Input: part model. Units: mm. Frame: model coordinates. A direction names the side the tool comes from. Give positions to 0.01 mm unless a question says otherwise; leave off trailing zeros. Write each loop counter-clockwise with the first axis right and the second up, starting at its lowest first coordinate (ties: lowest second). Pieces come first, ordered by that corner, then holes. Notation, with made-up numbers: (-29, -12.75) - (-1, -12.75) arc R34 cw to (-1, 21.25) - close; hole circle Ø4 at (10.5, 38). An arc over 180 degrees is marked (long way). Use a Markdown table: item, result. Add a question column.
1. Section query C-C, the plane y = -7. Return loops of the section in (x, z), plus the area to 3 significant figures.
2. Section query D-D, the plane x = -46. Return loops of the section in (y, z).
3. Pin query (flat end, axial travel): pin 1 (9.5 mm diameter, centred on x = -5, y = -6, fed in from +Z); pin 2 (10 mm diameter, centred on x = 0, z = -234.95, fed in from -Y). Return the tip coordinate at first contact, or that it passes through.
4. Material intervals for probe 1 along Z at (x, y) = (0, -16); probe 2 along Y at (x, z) = (-32, 244); probe 3 along Z at (x, y) = (12, -2), sorted ascending.
5. Mould query, pull axis X, two halves, no side actions, for faces 1 (the flat face through (-1, -19, -279.4)), 2 (the cylindrical face through (-1.38, -19.32, -241.15)), 3 (the flat face through (63.5, -19, -4)). Classes: released by +X, released by -X, zero draft, split by the parting line, or undercut.
6. Set-up query: faces 4 (the flat face through (-1, -9, 152.4)), 5 (the flat face through (-63.5, -19, -4)). Return all of +Z, -Z, +X, -X, +Y, -Y with unobstructed straight access to the full face (end or side cutting, diameter ignored); none if empty.
7. Section query A-A, the plane z = -234.95. Return loops of the section in (x, y).
8. Section query B-B, the plane x = 0. Return loops of the section in (y, z), plus the area to 3 significant figures.
```python
from build123d import *

# Parameters (mm, degrees)
F0_W     = 127
F0_H     = 558.8
F1_DEPTH = 38.1
F2_W     = 19.05
F2_H     = 127
F3_DEPTH = 152.4
F4_R     = 6.35
F5_DEPTH = 38.101


with BuildPart() as f1:
    # F0 (on Front) → F1 (new body)
    with BuildSketch(Plane.XZ):
        Rectangle(F0_W, F0_H)
    extrude(amount=F1_DEPTH)

    # F2 (on face) → F3 (cut)
    with BuildSketch(Plane(origin=(-63.5, 0, 0), x_dir=(0, -1, 0), z_dir=(-1, 0, 0))):
        with Locations((9.525, 215.9)):
            Rectangle(F2_W, F2_H)
    extrude(amount=-F3_DEPTH, mode=Mode.SUBTRACT)

    # F4 (on face) → F5 (cut, through all)
    with BuildSketch(Plane.XZ.offset(38.1)):
        with Locations((0, -234.95)):
            Circle(F4_R)
    extrude(amount=-F5_DEPTH, mode=Mode.SUBTRACT)


solid = f1.part
```
Result sheet:
| question | item | result |
|---|---|---|
| 1 | outline | (-63.5, -279.4) - (63.5, -279.4) - (63.5, 152.4) - (-63.5, 152.4) - close; hole circle Ø12.7 at (0, -234.95) |
| 1 | area | 54,700 mm² |
| 2 | outline | (-38.1, -279.4) - (0, -279.4) - (0, 152.4) - (-19.05, 152.4) - (-19.05, 279.4) - (-38.1, 279.4) - close |
| 3 | pin 1 | stops at z = 152.4 |
| 3 | pin 2 | passes through |
| 4 | probe 1 | z = -279.4 to -241.3, -228.6 to 152.4 |
| 4 | probe 2 | y = -38.1 to -19.05 |
| 4 | probe 3 | z = -279.4 to 152.4 |
| 5 | face 1 | zero draft |
| 5 | face 2 | undercut |
| 5 | face 3 | released by +X |
| 6 | face 4 | +Z, +X, -X, +Y |
| 6 | face 5 | +Z, -Z, -X, +Y, -Y |
| 7 | outline | (-63.5, -38.1) - (-6.35, -38.1) - (-6.35, 0) - (-63.5, 0) - close; (6.35, -38.1) - (63.5, -38.1) - (63.5, 0) - (6.35, 0) - close |
| 8 | outline | (-38.1, -279.4) - (0, -279.4) - (0, -241.3) - (-38.1, -241.3) - close; (-38.1, -228.6) - (0, -228.6) - (0, 152.4) - (-19.05, 152.4) - (-19.05, 279.4) - (-38.1, 279.4) - close |
| 8 | area | 18,400 mm² |
